Check sheet for the modelled part. Datum: model origin and axes. Units: mm. Round coordinates to 2 decimals unless told otherwise and drop trailing zeros. Loops run counter-clockwise (first coordinate to the right, second up) from the corner with the lowest first, then second, coordinate; pieces in that order, holes last. Notation, with made-up numbers: (60, 0) - (87, 0) arc R24 ccw to (87, 30) - close; hole circle Ø2 at (80.25, 10). An arc over 180 degrees is marked (long way). Put each result on its own line as item: value.
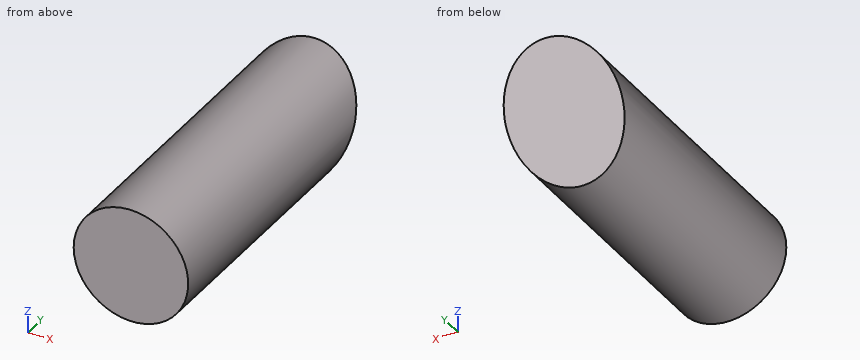
Autodesk Inventor part; units mm, degrees
ref_plane "YZ Plane" through (0, 0, 0) normal (1, 0, 0) x (0, 1, 0)
ref_plane "XZ Plane" through (0, 0, 0) normal (0, 1, 0) x (-1, 0, 0)
sketch "Sketch1" plane through (0, 0, 0) normal (0, 1, 0) x (-1, 0, 0)
  circle A0 centre (0, 0) radius 4
  dimension "d0" = 8
extrude "Extrusion1" add sketch "Sketch1" along normal blind 20
sketch "Sketch2" plane through (0, 20, 0) normal (0, 1, 0) x (1, 0, 0)
  circle A0 centre (0, 0) radius 4
  dimension "d3" = 8
extrude "Extrusion2" add sketch "Sketch2" along normal blind 2
sketch "Sketch3" plane through (0, 0, 0) normal (1, 0, 0) x (0, 1, 0)
  line L0 (22, -4) -> (22, 4)
  line L1 (22, 4) -> (17.3812, -4)
  line L2 (0, -4) -> (22, -4)
  line L3 (22, 4) -> (31.2376, 4) construction
  line L4 (17.3812, -4) -> (22, -4)
  line L5 (22, 4) -> (22, -4)
  point P0 (0, 0)
  dimension "d6" = 120
extrude "Extrusion3" cut sketch "Sketch3" along normal through all both and the other way through all
sketch "Sketch4" plane through (0, 0, 0) normal (1, 0, 0) x (0, 1, 0)
  point P0 (0, 0)
ref_plane "Work Plane2" through (0, 19.6906, 0) normal (0, 0.5, 0.866) x (-1, 0, 0)
ref_plane "Work Plane1" through (0, 19.6906, 0) normal (0, 0.866, 0.5) x (1, 0, 0)
properties part number "Camera encasing" material "Rubber"
Item 1: Thickness scan on line 1 (Z direction, x = 1, y = 15.75); line 2 (X direction, y = 8.5, z = 1.5); line 3 (Y direction, x = -2, z = -0.5). Record the ranges inside material, lowest first. Write a range as from..to.
Filled sheet:
line 1: -3.87..3.87
line 2: -3.71..3.71
line 3: 0..19.4
Item 2: Section check A-A on y = 17. Enter the section's corners in (x, z), then the cut area to 3 significant figures.
Filled sheet:
outline: circle Ø8 at (0, 0)
area: 50.3 mm²
Item 3: Section check B-B on z = 3. Enter the section's corners in (x, y), then the cut area to 3 significant figures.
Filled sheet:
outline: (-2.65, 0) - (2.65, 0) - (2.65, 21.42) - (-2.65, 21.42) - close
area: 113 mm²
Item 4: Go/stop test with flat-tipped pins: pin 1 (1 mm diameter, centred on x = -1, y = 18, fed in from -Z); pin 2 (1.5 mm diameter, centred on x = 0, z = 3, fed in from +Y); pin 3 (3 mm diameter, centred on x = -2, z = -2, fed in from +Y). Record where each tip stops, or that it passes through.
Filled sheet:
pin 1: z = -3.79
pin 2: y = 21.86
pin 3: y = 19.4
Item 5: Section check C-C on x = -0.5. Enter the section's corners in (y, z), then the cut area to 3 significant figures.
Filled sheet:
outline: (0, -3.97) - (17.4, -3.97) - (21.98, 3.97) - (0, 3.97) - close
area: 156 mm²
